For this review, take the finished solid that the model builds, in its own axes (mm). A direction names the side the tool comes from. Round coordinates to 2 decimals unless told otherwise and drop trailing zeros. Order: outer loops, then holes, each group sorted by start corner. A loop starts at its lowest first (then second) coordinate and runs counter-clockwise, first axis right, second up. Notation, with made-up numbers: (-34.5, 62) -> (1.5, 62) arc R26 cw to (1.5, 88) -> close; hole circle Ø9 at (0, -26). An arc over 180 degrees is marked (long way). Use a Markdown table: item, result. Add a question column.
1) Consider section C-C (z = 8). State the section outline as (x, y) points, plus the area to 3 significant figures.
2) Consider section A-A (y = 0). State the section outline as (x, z) points, plus the area to 3 significant figures.
3) Consider section D-D (z = 3.25). State the section outline as (x, y) points.
4) Draft analysis for pull direction X (two halves, no side actions). For faces 1 (the face through (0, 0, 0)), 2 (the face through (13.17, 20.66, 7.46)), 3 (the face through (-2.994, 22.804, 8.204)), state which applies: pulls with the +X half, pulls with the -X half, needs draft (parallel to the pull), parting line crosses it, or undercut.
5) Wall thickness on line 1 along X through (y, z) = (0.5, 9); line 2 along Y through (x, z) = (0, 7.5); line 3 along Z through (x, y) = (-15, 3): over which ranges is each line inside the solid? List them lowest first. Write a range as [from, to].
6) Machinability: for faces 4 (the face through (0, 0, 1.5)), 5 (the face through (-17.5, 17.5, 10)), 6 (the face through (-20.633, -15.821, 10.74)), which of the approach directions +Z, -Z, +X, -X, +Y, -Y give a long, thin tool a straight path to every point of the face, cutting with its end or side? Answer none if there is none.
7) Clearance check with flat-ended pins moving along their axes: P1, Ø6, axis at x = 0.5, z = 3.5, coming from the -Y side; P2, Ø1, axis at x = 17.5, y = -20.5, coming from the +Z side; P3, Ø1, axis at x = -6.5, z = 7, coming from the +Y side; P4, Ø6, axis at x = -1, y = 9.5, coming from the +Z side. State where each tip first meets the part, or that it passes through.
```python
from build123d import *

# Parameters (mm, degrees)
SKETCH_R      = 24.5
PAD_DEPTH     = 10
FILLET_R      = 5
THICKNESS_T   = -1.5
SKETCH001_R   = 26
SKETCH001_R_2 = 23
PAD001_DEPTH  = 1.5


with BuildPart() as part:
    # Sketch → Pad (new body)
    with BuildSketch(Plane.XY):
        Circle(SKETCH_R)
    extrude(amount=PAD_DEPTH)

    # Fillet
    fillet_edges = [part.edges().sort_by_distance(p)[0] for p in [
        (-24.5, 0, 0),
    ]]
    fillet(fillet_edges, radius=FILLET_R)

    # Thickness
    thickness_openings = [part.faces().sort_by_distance(p)[0] for p in [
        (0, 0, 10),
    ]]
    offset(amount=THICKNESS_T, openings=thickness_openings)

    # Sketch001 → Pad001 (new body)
    with BuildSketch(Plane.XY.offset(10)):
        Circle(SKETCH001_R)
        Circle(SKETCH001_R_2, mode=Mode.SUBTRACT)
    extrude(amount=PAD001_DEPTH)


solid = part.part
```
Results list:
| question | item | result |
|---|---|---|
| 1 | outline | circle Ø49 at (0, 0); hole circle Ø46 at (0, 0) |
| 1 | area | 224 mm2 |
| 2 | outline | (-26, 10) -> (-24.5, 10) -> (-24.5, 5) arc R5 ccw to (-19.5, 0) -> (19.5, 0) arc R5 ccw to (24.5, 5) -> (24.5, 10) -> (26, 10) -> (26, 11.5) -> (23, 11.5) -> (23, 5) arc R3.5 cw to (19.5, 1.5) -> (-19.5, 1.5) arc R3.5 cw to (-23, 5) -> (-23, 11.5) -> (-26, 11.5) -> close |
| 2 | area | 103 mm2 |
| 3 | outline | circle Ø48.37 at (0, 0); hole circle Ø45.06 at (0, 0) |
| 4 | face 1 | needs draft |
| 4 | face 2 | parting line crosses it |
| 4 | face 3 | undercut |
| 5 | line 1 | [-24.49, -22.99], [22.99, 24.49] |
| 5 | line 2 | [-24.5, -23], [23, 24.5] |
| 5 | line 3 | [0, 1.5] |
| 6 | face 4 | +Z |
| 6 | face 5 | -Z |
| 6 | face 6 | +Z, -Z |
| 7 | P1 | y = -24.5 |
| 7 | P2 | through |
| 7 | P3 | y = 23.75 |
| 7 | P4 | z = 1.5 |
